```python
from build123d import *

# Parameters (mm, degrees)
F0_R     = 12.7
F1_DEPTH = 15.24
F3_DEPTH = 6.35
F4_R     = 5.08


with BuildPart() as f1:
    # F0 (on Front) → F1 (new body)
    with BuildSketch(Plane.XZ):
        with BuildLine():
            Line((19.05, 38.1), (-19.05, 38.1))
            ThreePointArc((-19.05, 38.1), (-32.520384, 32.520384), (-38.1, 19.05))
            Line((-38.1, 19.05), (-38.1, -50.8))
            Line((-38.1, -50.8), (38.1, -50.8))
            Line((38.1, -50.8), (38.1, 19.05))
            ThreePointArc((38.1, 19.05), (32.520384, 32.520384), (19.05, 38.1))
        make_face()
        Circle(F0_R, mode=Mode.SUBTRACT)
    extrude(amount=F1_DEPTH)

    # F2 (on Front) → F3 (join)
    with BuildSketch(Plane.XZ):
        with BuildLine():
            Line((25.4, -50.8), (25.4, 0))
            Line((25.4, 0), (12.7, 0))
            ThreePointArc((12.7, 0), (0, -12.7), (-12.7, 0))
            Line((-12.7, 0), (-25.4, 0))
            Line((-25.4, 0), (-25.4, -50.8))
            Line((-25.4, -50.8), (25.4, -50.8))
        make_face()
    extrude(amount=-F3_DEPTH)

    # F4
    f4_edges = [f1.edges().sort_by_distance(p)[0] for p in [
        (-38.1, -15.24, -15.875),
        (-32.520384, -15.24, 32.520384),
        (0, -15.24, 38.1),
        (32.520384, -15.24, 32.520384),
        (38.1, -15.24, -15.875),
        (0, -15.24, -50.8),
    ]]
    fillet(f4_edges, radius=F4_R)


solid = f1.part
```
For this review, take the finished solid that the model builds, in its own axes (mm). A direction names the side the tool comes from. Round coordinates to 2 decimals unless told otherwise and drop trailing zeros. Loops run counter-clockwise (first coordinate to the right, second up) from the corner with the lowest first, then second, coordinate; pieces in that order, holes last.
Q1. Machinability: for faces 1 (the face through (-19, 3, 0)), 2 (the face through (25.4, 3, -26)), 3 (the face through (-25.4, 3, -25)), which of the approach directions +Z, -Z, +X, -X, +Y, -Y give a long, thin tool a straight path to every point of the face, cutting with its end or side? Answer none if there is none.
Result sheet:
face 1: +Z, +X, -X, +Y
face 2: +Z, -Z, +X, +Y
face 3: +Z, -Z, -X, +Y
Q2. Mouldability with a two-part tool opening along Z and no side actions: class faces 4 (the face through (-1.653, -6.995, -12.592)), 5 (the face through (38.1, -5, -16)), 6 (the face through (0, -5, 38.1)) as +Z half, -Z half, draft (parallel to the pull), parting line (faces both ways), or undercut.
Result sheet:
face 4: undercut
face 5: draft
face 6: +Z half
Q3. Add section D-D on z = -41. Write out the cut boundary in (x, y), plus the area to 3 significant figures.
Result sheet:
outline: (-38.1, -10.16) arc R5.08 ccw to (-33.02, -15.24) - (33.02, -15.24) arc R5.08 ccw to (38.1, -10.16) - (38.1, 0) - (25.4, 0) - (25.4, 6.35) - (-25.4, 6.35) - (-25.4, 0) - (-38.1, 0) - close
area: 1,470 mm2
Q4. Add section B-B on x = 0. Write out the cut boundary in (y, z).
Result sheet:
outline: (-15.24, -45.72) arc R5.08 ccw to (-10.16, -50.8) - (6.35, -50.8) - (6.35, -12.7) - (-15.24, -12.7) - close; (-15.24, 12.7) - (0, 12.7) - (0, 38.1) - (-10.16, 38.1) arc R5.08 ccw to (-15.24, 33.02) - close
Q5. To check wall thickness, follow line 1 along X through (y, z) = (-8, 0); line 2 along Z through (x, y) = (0, -0.5); line 3 along Y through (x, z) = (-30, 19). State the ranges of each line that lie inside material, in increasing order.
Result sheet:
line 1: x = -38.1 to -12.7, 12.7 to 38.1
line 2: z = -50.8 to -12.7, 12.7 to 38.1
line 3: y = -15.24 to 0
Q6. Add section A-A on y = -8.5. Write out the cut boundary in (x, z), plus the area to 3 significant figures.
Result sheet:
outline: (-38.1, -50.8) - (38.1, -50.8) - (38.1, 19.05) arc R19.05 ccw to (19.05, 38.1) - (-19.05, 38.1) arc R19.05 ccw to (-38.1, 19.05) - close; hole circle Ø25.4 at (0, 0)
area: 6,110 mm2
Q7. Insertion check: pin 1 Ø10 at (x, y) = (26, -7.5) entering from +Z; pin 2 Ø3 at (x, y) = (-20, 4.5) entering from +Z; pin 3 Ø3 at (y, z) = (4.5, -36.5) entering from +X. Each pin has a flat end and moves straight along its axis. Give the tip position at first contact, or say it passes through.
Result sheet:
pin 1: stops at z = 38
pin 2: stops at z = 0
pin 3: stops at x = 25.4
Q8. Add section C-C on z = 5.5. Write out the cut boundary in (x, y).
Result sheet:
outline: (-38.1, -10.16) arc R5.08 ccw to (-33.02, -15.24) - (-11.45, -15.24) - (-11.45, 0) - (-38.1, 0) - close; (11.45, -15.24) - (33.02, -15.24) arc R5.08 ccw to (38.1, -10.16) - (38.1, 0) - (11.45, 0) - close
